from build123d import *

# Parameters (mm, degrees)
SKETCH_1_W          = 380
SKETCH_1_H          = 291
EXTRUDE_1_DEPTH     = 3
SKETCH_2_W          = 380
SKETCH_2_H          = 291
SKETCH_2_W_2        = 344
SKETCH_2_H_2        = 255
EXTRUDE_3_DEPTH     = 3
SKETCH_7_W          = 105
SKETCH_7_H          = 225
CUT_EXTRUDE_1_DEPTH = 3


with BuildPart() as part:
    # Эскиз1 → Бобышка-Вытянуть1 (new body)
    with BuildSketch(Plane(origin=(0, 0, 0), x_dir=(1, 0, 0), z_dir=(0, 1, 0))):
        Rectangle(SKETCH_1_W, SKETCH_1_H)
    extrude(amount=EXTRUDE_1_DEPTH)

    # Эскиз2 → Бобышка-Вытянуть3 (add)
    with BuildSketch(Plane.XZ):
        Rectangle(SKETCH_2_W, SKETCH_2_H)
        Rectangle(SKETCH_2_W_2, SKETCH_2_H_2, mode=Mode.SUBTRACT)
    extrude(amount=EXTRUDE_3_DEPTH)

    # Эскиз7 → Вырез-Вытянуть1 (cut)
    with BuildSketch(Plane.XZ):
        with Locations((119.5, 15)):
            Rectangle(SKETCH_7_W, SKETCH_7_H)
    extrude(amount=-CUT_EXTRUDE_1_DEPTH, mode=Mode.SUBTRACT)


solid = part.part
Geometry check sheet. Reference: the model listing, model coordinates, mm. Give positions to 0.01 mm unless a question says otherwise; leave off trailing zeros. Write each loop counter-clockwise with the first axis right and the second up, starting at its lowest first coordinate (ties: lowest second). Pieces come first, ordered by that corner, then holes. Notation, with made-up numbers: M 33,82 L 83,82 A25 cw 83,115 Z; hole C 20.25,39 d4. An arc over 180 degrees is marked long. Answer as CSV lines item,"result". Start each with the question number.
Q1. Section check D-D, the plane x = -2.5. Record the cut outline in (y, z).
Q2. Section check A-A, the plane z = 79. Record the cut outline in (x, y).
Q3. Section check C-C, the plane y = 0.9. Record the cut outline in (x, z), then the cut area to 3 significant figures.
Q4. Section check B-B, the plane x = 107.5. Record the cut outline in (y, z).
Q5. Material ranges on L1, parallel to X at y = 2.4, z = -64.5; L2, parallel to X at y = -0.35, z = 18.5; L3, parallel to Z at x = 46, y = -0.3, recorded low to high.
Q6. Release check for a two-part mould opening along Z. For faces 1 (the face through (-41, 0, -2)), 2 (the face through (-45, 3, -2)) record: pulls with the +Z half, pulls with the -Z half, needs draft (parallel to the pull), parting line crosses it, or undercut.
Q7. Go/stop test with a flat-tipped pin: pin 1 (3 mm diameter, centred on x = 34.5, z = 87.5, fed in from -Y). Record where the tip stops, or that it passes through.
Geometry says:
1,outline,"M -3,-145.5 L 3,-145.5 L 3,145.5 L -3,145.5 L -3,127.5 L 0,127.5 L 0,-127.5 L -3,-127.5 Z"
2,outline,"M -190,-3 L -172,-3 L -172,0 L 67,0 L 67,3 L -190,3 Z; M 172,-3 L 190,-3 L 190,3 L 172,3 Z"
3,outline,"M -190,-145.5 L 190,-145.5 L 190,145.5 L -190,145.5 Z; hole M 67,-97.5 L 172,-97.5 L 172,127.5 L 67,127.5 Z"
3,area,"87,000 mm^2"
4,outline,"M -3,-145.5 L 3,-145.5 L 3,-97.5 L 0,-97.5 L 0,-127.5 L -3,-127.5 Z; M -3,127.5 L 3,127.5 L 3,145.5 L -3,145.5 Z"
5,L1,"-190 to 67, 172 to 190"
5,L2,"-190 to -172, 172 to 190"
5,L3,"-145.5 to -127.5, 127.5 to 145.5"
6,face 1,"undercut"
6,face 2,"needs draft"
7,pin 1,"y = 0"
